Verification items for the finished model (mm, model axes). A direction names the side the tool comes from. Give positions to 0.01 mm unless a question says otherwise; leave off trailing zeros. Order: outer loops, then holes, each group sorted by start corner. A loop starts at its lowest first (then second) coordinate and runs counter-clockwise, first axis right, second up. Notation, with made-up numbers: (44.5, 16.5) - (98.5, 16.5) arc R9 ccw to (98.5, 29.5) - close; hole circle Ø5 at (-13.5, 15). An arc over 180 degrees is marked (long way). Answer as a JSON object with one key per item and string values. Group by question number.
(1) Depth check by flat-ended pin: pin 1 Ø2.5 at (x, y) = (-25, 0) entering from -Z; pin 2 Ø5 at (x, y) = (25, 0) entering from -Z; pin 3 Ø1.5 at (x, z) = (-8, 2.5) entering from +Y; pin 4 Ø2 at (x, z) = (49, 3) entering from +Y. Enter the tip coordinate at first touch or a pass-through.
(2) Section check C-C (z = 2.9). Record the boundary of the cut face in (x, y) (1 decimal).
(3) Access from +Z, -Z, +X, -X, +Y, -Y to the whole of each face (thin tool, end or side, straight path). Record for faces 4 (the face through (5, 7.5, 2)), 5 (the face through (66.242, 25, 2)).
(4) Section check B-B (y = 0). Record the boundary of the cut face in (x, z).
(5) Mould release check, pull along Y, two halves, no side actions. Record for faces 1 (the face through (18, 4, 0)), 2 (the face through (64.58, 27.76, 2.46)), 3 (the face through (4, -7.5, 2)): +Y half, -Y half, draft (parallel to the pull), parting line (faces both ways), or undercut.
(6) Section check D-D (x = 1.5). Record the boundary of the cut face in (y, z).
(7) Thickness scan on line 1 (Y direction, x = 25, z = 3.5); line 2 (X direction, y = 0.5, z = 3.8); line 3 (Y direction, x = 61.5, z = 3.1) (3 decimals). Record the ranges inside material, lowest first.
(8) Section check A-A (x = 25). Record the boundary of the cut face in (y, z).
Autodesk Inventor part; units mm, degrees
ref_plane "YZ Plane" through (0, 0, 0) normal (1, 0, 0) x (0, 1, 0)
ref_plane "XZ Plane" through (0, 0, 0) normal (0, 1, 0) x (-1, 0, 0)
ref_plane "XY Plane" through (0, 0, 0) normal (0, 0, 1) x (1, 0, 0)
ref_plane "Work Plane1" through (0, 0, 0) normal (0, 0, 1) x (1, 0, 0)
sketch "Sketch1" plane through (0, 0, 0) normal (0, 0, 1) x (1, 0, 0)
  line L0 (28, 30) -> (30, 28) construction
  line L1 (28, 30) -> (-28, 30) construction
  line L2 (-30, 28) -> (-28, 30) construction
  line L3 (-30, 28) -> (-30, -28) construction
  line L4 (-28, -30) -> (-30, -28) construction
  line L5 (-28, -30) -> (28, -30) construction
  line L6 (30, -28) -> (28, -30) construction
  line L7 (30, -28) -> (30, 28) construction
  circle A0 centre (25, 0) radius 1.3 construction
  circle A1 centre (-25, 0) radius 1.3 construction
  circle A2 centre (0, 0) radius 7.5 construction
  line L8 (-30, -7.5) -> (40, -7.5)
  line L9 (40, -7.5) -> (40, 7.5)
  line L10 (40, 7.5) -> (-30, 7.5)
  line L11 (-30, 7.5) -> (-30, -7.5)
  line L12 (40, -7.5) -> (66.2425, 18.7425)
  line L13 (40, -7.5) -> (77.1125, -7.5) construction
  line L14 (66.2425, 18.7425) -> (66.2425, 27.2511)
  line L15 (40, 7.5) -> (56.2425, 23.7425)
  line L16 (40, 7.5) -> (62.9703, 7.5) construction
  line L17 (56.2425, 23.7425) -> (56.2425, 27.2511)
  line L18 (66.2425, 27.2511) -> (66.2425, 33.815)
  line L19 (66.2425, 33.815) -> (56.2425, 33.815)
  line L20 (56.2425, 33.815) -> (56.2425, 27.2511)
  circle A3 centre (-25, 0) radius 2
  circle A4 centre (25, 0) radius 2
  circle A5 centre (61.2425, 28.815) radius 3.5
  line L21 (79.415, 27.3813) -> (49.415, 27.3813) construction
  line L22 (79.415, 30.2423) -> (49.415, 30.2423) construction
  line L23 (62.6454, 27.3813) -> (62.6454, -21.1882) construction
  line L24 (59.7845, 27.3813) -> (59.7845, -21.1882) construction
  point P0 (0, 0)
  dimension "d0" = 70
  dimension "d1" = 45
  dimension "d2" = 45
  dimension "d3" = 10
  dimension "d4" = 15
  dimension "d5" = 7.5
  dimension "d7" = 4
  dimension "d8" = 4
  dimension "d11" = 7
  dimension "d12" = 5
  dimension "d13" = 5
extrude "Extrusion1" add sketch "Sketch1" along normal blind 5
fillet "Fillet1" radius 4 6 edges at (40, 7.5, 2.5) (56.2425, 33.815, 2.5) (66.2425, 33.815, 2.5) (66.2425, 18.7425, 2.5) (40, -7.5, 2.5) (56.2425, 23.7425, 2.5)
properties part number "10_MiniSPIM_Sampleholder"
Solutions:
{
 "1": {"pin 1": "passes through", "pin 2": "stops at z = 0", "pin 3": "stops at y = 7.5", "pin 4": "stops at y = 17.5"},
 "2": {"outline": "(-30, -7.5) - (38.3, -7.5) arc R4 ccw to (41.2, -6.3) - (65.1, 17.6) arc R4 ccw to (66.2, 20.4) - (66.2, 29.8) arc R4 ccw to (62.2, 33.8) - (60.2, 33.8) arc R4 ccw to (56.2, 29.8) - (56.2, 25.4) arc R4 cw to (55.1, 22.6) - (41.2, 8.7) arc R4 cw to (38.3, 7.5) - (-30, 7.5) - close; hole circle Ø4 at (-25, 0); hole circle Ø4 at (25, 0); hole circle Ø7 at (61.2, 28.8)"},
 "3": {"face 4": "+Z, -Z, -X, +Y", "face 5": "+Z, -Z, +X, +Y, -Y"},
 "4": {"outline": "(-30, 0) - (-27, 0) - (-27, 5) - (-30, 5) - close; (-23, 0) - (23, 0) - (23, 5) - (-23, 5) - close; (27, 0) - (47.5, 0) - (47.5, 5) - (27, 5) - close"},
 "5": {"face 1": "draft", "face 2": "undercut", "face 3": "-Y half"},
 "6": {"outline": "(-7.5, 0) - (7.5, 0) - (7.5, 5) - (-7.5, 5) - close"},
 "7": {"line 1": "y = -7.5 to -2, 2 to 7.5", "line 2": "x = -30 to -26.94, -23.06 to 23.06, 26.94 to 48", "line 3": "y = 14 to 25.324, 32.306 to 33.815"},
 "8": {"outline": "(-7.5, 0) - (-2, 0) - (-2, 5) - (-7.5, 5) - close; (2, 0) - (7.5, 0) - (7.5, 5) - (2, 5) - close"}
}
